Verification items for the finished model (mm, model axes). A direction names the side the tool comes from. Round coordinates to 2 decimals unless told otherwise and drop trailing zeros. Loops run counter-clockwise (first coordinate to the right, second up) from the corner with the lowest first, then second, coordinate; pieces in that order, holes last. Notation, with made-up numbers: M -9,88 L 29,88 A25 ccw 29,127 Z; hole C 57.5,-12.75 d4. An arc over 180 degrees is marked long. One line per item, written item: value.
from build123d import *

# Parameters (mm, degrees)
F1_DEPTH  = 65
F3_R      = 5
F4_DEPTH  = 4
F7_DEPTH  = 25
F8_R      = 1
F10_DEPTH = 4.001


with BuildPart() as f1:
    # F0 (on Top) → F1 (new body)
    with BuildSketch(Plane.XY):
        with BuildLine():
            Line((-71.158341, -41.139144), (-71.158341, -45.139144))
            Line((-71.158341, -45.139144), (45.970776, -45.139144))
            ThreePointArc((45.970776, -45.139144), (53.041844, -42.210212), (55.970776, -35.139144))
            Line((55.970776, -35.139144), (55.970776, 5.481472))
            ThreePointArc((55.970776, 5.481472), (53.041844, 12.552539), (45.970776, 15.481472))
            Line((45.970776, 15.481472), (30.353561, 15.481472))
            Line((30.353561, 15.481472), (30.353561, 11.481472))
            Line((30.353561, 11.481472), (45.970776, 11.481472))
            ThreePointArc((45.970776, 11.481472), (50.213417, 9.724112), (51.970776, 5.481472))
            Line((51.970776, 5.481472), (51.970776, -35.139144))
            ThreePointArc((51.970776, -35.139144), (50.213417, -39.381785), (45.970776, -41.139144))
            Line((45.970776, -41.139144), (-71.158341, -41.139144))
        make_face()
    extrude(amount=F1_DEPTH)

    # F3 (on face) → F4 (cut)
    with BuildSketch(Plane(origin=(0, 15.481472, 0), x_dir=(-1, 0, 0), z_dir=(0, 1, 0))):
        with Locations((-36.970776, 10)):
            Circle(F3_R)
        with Locations((-36.970776, 55)):
            Circle(F3_R)
    extrude(amount=-F4_DEPTH, mode=Mode.SUBTRACT)

    # F6 (on face) → F7 (cut)
    with BuildSketch(Plane(origin=(0, -41.139144, 0), x_dir=(-1, 0, 0), z_dir=(0, 1, 0))):
        with BuildLine():
            Line((78.911833, 65.031889), (61.355465, 65.031889))
            ThreePointArc((61.355465, 65.031889), (37.238592, 32.5), (61.355465, -0.031889))
            Line((61.355465, -0.031889), (78.911833, -0.031889))
            Line((78.911833, -0.031889), (78.911833, 65.031889))
        make_face()
    extrude(amount=-F7_DEPTH, mode=Mode.SUBTRACT)

    # F8
    f8_edges = [f1.edges().sort_by_distance(p)[0] for p in [
        (-61.2511, -43.139144, 65),
        (-61.2511, -43.139144, 0),
    ]]
    fillet(f8_edges, radius=F8_R)

    # F9 (on face) → F10 (cut, through all)
    with BuildSketch(Plane(origin=(0, -41.139144, 0), x_dir=(-1, 0, 0), z_dir=(0, 1, 0))):
        with BuildLine():
            Line((-39.483187, 26.849984), (-30.483187, 26.849984))
            ThreePointArc((-30.483187, 26.849984), (-24.983187, 32.349983), (-30.483186, 37.849984))
            Line((-30.483186, 37.849984), (-39.483187, 37.849984))
            ThreePointArc((-39.483187, 37.849984), (-44.983187, 32.349984), (-39.483187, 26.849984))
        make_face()
    extrude(amount=-F10_DEPTH, mode=Mode.SUBTRACT)


solid = f1.part
(1) Sectioned sample at B-B on x = -44.5. Enter the section's corners in (y, z).
Completed:
outline: M -45.14,0 L -41.14,0 L -41.14,11.5 L -45.14,11.5 Z; M -45.14,53.5 L -41.14,53.5 L -41.14,65 L -45.14,65 Z
(2) Sectioned sample at D-D on z = 31. Enter the section's corners in (x, y).
Completed:
outline: M -37.27,-45.14 L 25.15,-45.14 L 25.15,-41.14 L -37.27,-41.14 Z; M 30.35,11.48 L 45.97,11.48 A6 cw 51.97,5.48 L 51.97,-35.14 A6 cw 45.97,-41.14 L 44.81,-41.14 L 44.81,-45.14 L 45.97,-45.14 A10 ccw 55.97,-35.14 L 55.97,5.48 A10 ccw 45.97,15.48 L 30.35,15.48 Z
(3) Depth check by flat-ended pin: pin 1 Ø1.5 at (x, z) = (-36.5, 57) entering from +Y; pin 2 Ø1 at (y, z) = (-2, 44.5) entering from -X; pin 3 Ø1.2 at (y, z) = (14, 40.5) entering from -X. Enter the tip coordinate at first touch or a pass-through.
Completed:
pin 1: stops at y = -41.14
pin 2: stops at x = 51.97
pin 3: stops at x = 30.35
(4) Sectioned sample at A-A on z = 57. Enter the section's corners in (x, y), and give its area (3 significant figures).
Completed:
outline: M -47.66,-45.14 L 45.97,-45.14 A10 ccw 55.97,-35.14 L 55.97,5.48 A10 ccw 45.97,15.48 L 41.55,15.48 L 41.55,11.48 L 45.97,11.48 A6 cw 51.97,5.48 L 51.97,-35.14 A6 cw 45.97,-41.14 L -47.66,-41.14 Z; M 30.35,11.48 L 32.39,11.48 L 32.39,15.48 L 30.35,15.48 Z
area: 663 mm^2
(5) Thickness scan on L1, parallel to Y at x = 45.5, z = 8.5; L2, parallel to Y at x = -10, z = 8; L3, parallel to Y at x = 47, z = 54. Record the ranges inside material, lowest first. Write a range as from..to.
Completed:
L1: y = -45.14..-41.14, 11.48..15.48
L2: y = -45.14..-41.14
L3: y = -45.09..-41.05, 11.39..15.43
(6) Mould release check, pull along X, two halves, no side actions. Record for faces 1 (the face through (35, -43, 26.85)), 2 (the face through (24.985, -43.111, 32.229)), 3 (the face through (30.354, 14, 32)), 4 (the face through (38, 11.481, 32)): +X half, -X half, draft (parallel to the pull), parting line (faces both ways), or undercut.
Completed:
face 1: undercut
face 2: undercut
face 3: -X half
face 4: draft
(7) Tool access check on faces 5 (the face through (40.656, 13.509, 13.379)), 6 (the face through (-37.243, -43.111, 33.033)), 7 (the face through (50.167, 9.771, 32.045)), 8 (the face through (35, -43, 37.85)), 9 (the face through (16, -42, 65)). Record the directions out of +Z, -Z, +X, -X, +Y, -Y that give a thin tool (end or side, any length) a straight path to the whole face; none if there is none.
Completed:
face 5: +Y
face 6: -X, +Y, -Y
face 7: +Z, -Z, -X
face 8: -Y
face 9: +Z, +X, -X, +Y, -Y
(8) Sectioned sample at C-C on y = -27.5. Enter the section's corners in (x, z), and give its area (3 significant figures).
Completed:
outline: M 51.97,0 L 55.97,0 L 55.97,65 L 51.97,65 Z
area: 260 mm^2
